Source: CAD feature listing. Evaluate the final solid. Frame: model axes, mm. A direction names the side the tool comes from. Round coordinates to 2 decimals unless told otherwise and drop trailing zeros. Order: outer loops, then holes, each group sorted by start corner. A loop starts at its lowest first (then second) coordinate and runs counter-clockwise, first axis right, second up. Notation, with made-up numbers: (14, -34) - (25, -34) arc R25 cw to (25, -11) - close; hole circle Ø8 at (-5.5, -18.75). An arc over 180 degrees is marked (long way). Put each result on its own line as item: value. Start each with the question number.
1) Contact query for flat-ended pins moving along their axis: P1, Ø4, axis at x = -21, z = 8.5, coming from the +Y side; P2, Ø1, axis at x = 0, z = 7, coming from the +Y side; P3, Ø3, axis at y = 7.5, z = 2.5, coming from the +X side. Output: stop coordinate, or through.
2) Mould query, pull axis X, two halves, no side actions, for faces 6 (the face through (-4.99, -22.08, 6.26)), 7 (the face through (1.97, 20.68, 6.26)), 8 (the face through (19.031, -8.868, 6.261)). Classes: +X half, -X half, draft (parallel to the pull), parting line (faces both ways), or undercut.
3) Access query for faces 1 (the face through (-14.05, 15.3, 6.26)), 2 (the face through (-21, -4.012, 6)), 3 (the face through (21.615, 6.721, 6.261)), 4 (the face through (18.935, 2.089, 6.261)), 5 (the face through (-19.056, 8.264, 6.261)). Directions: +Z, -Z, +X, -X, +Y, -Y. A direction counts if a zero-diameter tool reaches every point of the face in a straight line with its end or side. Return the directions, or none.
4) Line query: probe 1 along X at (y, z) = (2.5, 7.75); probe 2 along Y at (x, z) = (-17.5, 7.5); probe 3 along Y at (x, z) = (19.5, 9). Output: solid intervals per line, ascending. Write a range as [from, to].
5) Section A-A on x = -0.5. Output: boundary loops of the cut face in (y, z).
6) Section C-C on y = 12.5. Output: boundary loops of the cut face in (x, z), then the cut area to 3 significant figures.
7) Section B-B on x = -13.5. Output: boundary loops of the cut face in (y, z), then the cut area to 3 significant figures.
```python
from build123d import *

# Parameters (mm, degrees)
EXTRUSION3_DEPTH = 12.7


with BuildPart() as part:
    # Sketch1 → Extrusion3 (new body)
    with BuildSketch(Plane.XY):
        with BuildLine():
            Line((21.213296498, 8.610485701), (17.381714073, 7.796057715))
            ThreePointArc((17.381714073, 7.796057715), (16.433889851, 9.634820412), (15.292273906, 11.359967376))
            Line((15.292273906, 11.359967376), (18.116572419, 13.411940358))
            Line((18.116572419, 13.411940358), (15.877110608, 16.494295106))
            Line((15.877110608, 16.494295106), (12.708043593, 14.191833146))
            ThreePointArc((12.708043593, 14.191833146), (11.094270913, 15.486111613), (9.349672368, 16.597774749))
            Line((9.349672368, 16.597774749), (11.095184843, 19.621091042))
            Line((11.095184843, 19.621091042), (7.795628055, 21.526091042))
            Line((7.795628055, 21.526091042), (5.837036927, 18.133711697))
            ThreePointArc((5.837036927, 18.133711697), (-11.299849109, 15.336750311), (-19.048930763, -0.201833587))
            Line((-19.048930763, -0.201833587), (-22.539955714, -0.201833587))
            Line((-22.539955714, -0.201833587), (-22.539955714, -4.011833587))
            Line((-22.539955714, -4.011833587), (-18.622773458, -4.011833587))
            ThreePointArc((-18.622773458, -4.011833587), (-18.077961731, -6.007478644), (-17.319971056, -7.932282309))
            Line((-17.319971056, -7.932282309), (-20.509181042, -9.352210079))
            Line((-20.509181042, -9.352210079), (-18.959514432, -12.832818272))
            Line((-18.959514432, -12.832818272), (-15.380990376, -11.239556711))
            ThreePointArc((-15.380990376, -11.239556711), (-14.071578126, -12.841074295), (-12.596231006, -14.291167358))
            Line((-12.596231006, -14.291167358), (-14.932182648, -16.885504485))
            Line((-14.932182648, -16.885504485), (-12.100800863, -19.434892096))
            Line((-12.100800863, -19.434892096), (-9.479694325, -16.523858372))
            ThreePointArc((-9.479694325, -16.523858372), (-7.632090826, -17.454331543), (-5.694488182, -18.178979739))
            Line((-5.694488182, -18.178979739), (-6.77327422, -21.499141767))
            Line((-6.77327422, -21.499141767), (-3.149748893, -22.676496515))
            Line((-3.149748893, -22.676496515), (-1.939273006, -18.951034806))
            ThreePointArc((-1.939273006, -18.951034806), (0.127054312, -19.0495763), (2.191883381, -18.923481372))
            Line((2.191883381, -18.923481372), (2.556794854, -22.395382123))
            Line((2.556794854, -22.395382123), (6.345923276, -21.997128678))
            Line((6.345923276, -21.997128678), (5.936466234, -18.101405157))
            ThreePointArc((5.936466234, -18.101405157), (7.864230606, -17.350976254), (9.699258395, -16.395941162))
            Line((9.699258395, -16.395941162), (11.44477087, -19.419257455))
            Line((11.44477087, -19.419257455), (14.744327659, -17.514257455))
            Line((14.744327659, -17.514257455), (12.785736531, -14.12187811))
            ThreePointArc((12.785736531, -14.12187811), (14.241609984, -12.652234785), (15.529543518, -11.033393772))
            Line((15.529543518, -11.033393772), (18.353842031, -13.085366754))
            Line((18.353842031, -13.085366754), (20.593303842, -10.003012005))
            Line((20.593303842, -10.003012005), (17.424236827, -7.700550045))
            ThreePointArc((17.424236827, -7.700550045), (18.156485614, -5.76580698), (18.674629484, -3.763072364))
            Line((18.674629484, -3.763072364), (22.089367164, -4.488897265))
            Line((22.089367164, -4.488897265), (22.881510706, -0.762154906))
            Line((22.881510706, -0.762154906), (19.049928281, 0.05227308))
            ThreePointArc((19.049928281, 0.05227308), (18.931939936, 2.117581232), (18.59070236, 4.157918442))
            Line((18.59070236, 4.157918442), (22.00544004, 4.883743342))
            Line((22.00544004, 4.883743342), (21.213296498, 8.610485701))
        make_face()
        with BuildLine():
            Line((-3.343536182, 3.146775418), (-2.067167627, 2.409863689))
            ThreePointArc((-2.067167627, 2.409863689), (0.010648283, 3.174982144), (2.083285387, 2.395943863))
            Line((2.083285387, 2.395943863), (3.353593084, 3.129356353))
            Line((3.353593084, 3.129356353), (4.396955543, 1.322199563))
            Line((4.396955543, 1.322199563), (3.120586988, 0.585287835))
            ThreePointArc((3.120586988, 0.585287835), (2.744291052, -1.596712756), (1.033305558, -3.00215))
            Line((1.033305558, -3.00215), (1.033305558, -4.468974981))
            Line((1.033305558, -4.468974981), (-1.053419361, -4.468974981))
            Line((-1.053419361, -4.468974981), (-1.053419361, -2.995151524))
            ThreePointArc((-1.053419361, -2.995151524), (-2.754939335, -1.578269388), (-3.116590945, 0.606206137))
            Line((-3.116590945, 0.606206137), (-4.386898641, 1.339618628))
            Line((-4.386898641, 1.339618628), (-3.343536182, 3.146775418))
        make_face(mode=Mode.SUBTRACT)
        with BuildLine():
            Line((-1.63378941, 22.835830278), (-2.043246451, 18.940106756))
            ThreePointArc((-2.043246451, 18.940106756), (-0.127054312, 19.0495763), (1.790427538, 18.965676082))
            Line((1.790427538, 18.965676082), (2.155339011, 22.437576832))
            Line((2.155339011, 22.437576832), (-1.63378941, 22.835830278))
        make_face()
        with BuildLine():
            Line((-10.780709843, 20.197047001), (-9.570233956, 16.471585292))
            ThreePointArc((-9.570233956, 16.471585292), (-7.864230606, 17.350976254), (-6.078398478, 18.054239722))
            Line((-6.078398478, 18.054239722), (-7.157184516, 21.37440175))
            Line((-7.157184516, 21.37440175), (-10.780709843, 20.197047001))
        make_face()
        with BuildLine():
            Line((-18.063547605, 14.066010814), (-15.442441067, 11.154977091))
            ThreePointArc((-15.442441067, 11.154977091), (-14.241609984, 12.652234785), (-12.896214177, 14.021061297))
            Line((-12.896214177, 14.021061297), (-15.23216582, 16.615398425))
            Line((-15.23216582, 16.615398425), (-18.063547605, 14.066010814))
        make_face()
        with BuildLine():
            Line((-22.223033883, 5.502833572), (-18.644509827, 3.909572011))
            ThreePointArc((-18.644509827, 3.909572011), (-18.156485614, 5.76580698), (-17.484157287, 7.563513996))
            Line((-17.484157287, 7.563513996), (-20.673367273, 8.983441766))
            Line((-20.673367273, 8.983441766), (-22.223033883, 5.502833572))
        make_face()
    extrude(amount=EXTRUSION3_DEPTH)


solid = part.part
```
Answer sheet:
1. P1: y = 8.98
1. P2: y = 22.72
1. P3: x = 21.77
2. face 6: -X half
2. face 7: undercut
2. face 8: +X half
3. face 1: +Z, -Z, +Y
3. face 2: +Z, -Z, -X
3. face 3: +Z, -Z, +X, +Y
3. face 4: +Z, -Z, +X
3. face 5: +Z, -Z
4. probe 1: [-18.89, -3.72], [-2.22, -1.96], [1.96, 2.26], [3.72, 18.89]
4. probe 2: [-12.18, -8.01], [-7.53, 7.57], [13.44, 14.57]
4. probe 3: [-11.51, -9.21], [-3.94, -0.04], [4.35, 8.25]
5. outline: (-19.04, 0) - (-4.47, 0) - (-4.47, 12.7) - (-19.04, 12.7) - close; (3.14, 0) - (22.72, 0) - (22.72, 12.7) - (3.14, 12.7) - close
6. outline: (-16.65, 0) - (16.86, 0) - (16.86, 12.7) - (-16.65, 12.7) - close
6. area: 426 mm^2
7. outline: (-18.18, 0) - (-15.29, 0) - (-15.29, 12.7) - (-18.18, 12.7) - close; (-13.44, 0) - (14.69, 0) - (14.69, 12.7) - (-13.44, 12.7) - close
7. area: 394 mm^2
